```python
from build123d import *

# Parameters (mm, degrees)
SKETCH1_W           = 120
SKETCH1_H           = 120
BOSS_EXTRUDE1_DEPTH = 60
SHELL1_T            = -2
FILLET1_R           = 2
CUT_EXTRUDE1_REACH  = 148.969
SKETCH2_W           = 15
SKETCH2_H           = 15


with BuildPart() as part:
    # Sketch1 → Boss-Extrude1 (new body)
    with BuildSketch(Plane(origin=(0, 0, 0), x_dir=(1, 0, 0), z_dir=(0, 1, 0))):
        Rectangle(SKETCH1_W, SKETCH1_H)
    extrude(amount=BOSS_EXTRUDE1_DEPTH)

    # Shell1
    shell1_openings = [part.faces().sort_by_distance(p)[0] for p in [
        (0, 60, 0),
    ]]
    offset(amount=SHELL1_T, openings=shell1_openings, kind=Kind.INTERSECTION)

    # Fillet1
    fillet1_edges = [part.edges().sort_by_distance(p)[0] for p in [
        (0, 0, 60),
        (-60, 0, 0),
        (0, 0, -60),
        (60, 0, 0),
        (60, 30, 60),
        (-60, 30, 60),
        (-60, 30, -60),
        (60, 30, -60),
    ]]
    fillet(fillet1_edges, radius=FILLET1_R)

    # Sketch2 → Cut-Extrude1 (cut, up to next)
    with BuildSketch(Plane.XY.offset(60), mode=Mode.PRIVATE) as cut_extrude1_sk1:
        with Locations((-12.5, 25)):
            Rectangle(SKETCH2_W, SKETCH2_H)
    cut_extrude1_tool1 = extrude(cut_extrude1_sk1.sketch, amount=-CUT_EXTRUDE1_REACH, mode=Mode.PRIVATE) & part.part
    # Sketch2 → Cut-Extrude1 (cut, up to next)
    with BuildSketch(Plane.XY.offset(60), mode=Mode.PRIVATE) as cut_extrude1_sk2:
        with Locations((12.5, 25)):
            Rectangle(SKETCH2_W, SKETCH2_H)
    cut_extrude1_tool2 = extrude(cut_extrude1_sk2.sketch, amount=-CUT_EXTRUDE1_REACH, mode=Mode.PRIVATE) & part.part
    add(cut_extrude1_tool1.solids().sort_by_distance((-12.5, 25, 60))[0], mode=Mode.SUBTRACT)
    add(cut_extrude1_tool2.solids().sort_by_distance((12.5, 25, 60))[0], mode=Mode.SUBTRACT)


solid = part.part
```
Part model, mm, in its own coordinate system. A direction names the side the tool comes from. Round coordinates to 2 decimals unless told otherwise and drop trailing zeros. Loops run counter-clockwise (first coordinate to the right, second up) from the corner with the lowest first, then second, coordinate; pieces in that order, holes last. Notation, with made-up numbers: (20, 21.25) -> (52, 21.25) arc R10 cw to (52, 27.25) -> close; hole circle Ø10 at (61, 44). An arc over 180 degrees is marked (long way). Use a Markdown table: item, result.
1) Cut at A-A, the plane y = 40.5. List the corners of the cut face in (x, z), and give its area (3 significant figures).
The answers:
| item | result |
|---|---|
| outline | (-60, -58) arc R2 ccw to (-58, -60) -> (58, -60) arc R2 ccw to (60, -58) -> (60, 58) arc R2 ccw to (58, 60) -> (-58, 60) arc R2 ccw to (-60, 58) -> close; hole (-58, -58) -> (58, -58) -> (58, 58) -> (-58, 58) -> close |
| area | 941 mm2 |
2) Drop flat-ended pins along their axis: pin 1 Ø4 at (x, z) = (-32, -5.5) entering from +Y; pin 2 Ø1 at (x, y) = (11.5, 23.5) entering from +Z; pin 3 Ø0.6 at (x, z) = (-15.5, 59) entering from -Y. Give the stop position or say it passes through.
The answers:
| item | result |
|---|---|
| pin 1 | stops at y = 2 |
| pin 2 | stops at z = -58 |
| pin 3 | stops at y = 0.13 |
3) Cut at B-B, the plane x = -18. List the corners of the cut face in (y, z).
The answers:
| item | result |
|---|---|
| outline | (0, -58) arc R2 ccw to (2, -60) -> (60, -60) -> (60, -58) -> (2, -58) -> (2, 58) -> (17.5, 58) -> (17.5, 60) -> (2, 60) arc R2 ccw to (0, 58) -> close; (32.5, 58) -> (60, 58) -> (60, 60) -> (32.5, 60) -> close |
4) Pull direction Z, two halves, no side cores. Call faces 3 (the flat face through (-1, 31, -60)), 4 (the flat face through (-1, 2, -1)), 5 (the flat face through (-60, 31, 1)), 6 (the flat face through (-1, 31, 60)): pulls with the +Z half, pulls with the -Z half, needs draft (parallel to the pull), parting line crosses it, or undercut.
The answers:
| item | result |
|---|---|
| face 3 | pulls with the -Z half |
| face 4 | undercut |
| face 5 | needs draft |
| face 6 | pulls with the +Z half |
5) Cut at C-C, the plane x = -49. List the corners of the cut face in (y, z).
The answers:
| item | result |
|---|---|
| outline | (0, -58) arc R2 ccw to (2, -60) -> (60, -60) -> (60, -58) -> (2, -58) -> (2, 58) -> (60, 58) -> (60, 60) -> (2, 60) arc R2 ccw to (0, 58) -> close |
6) Probe line 1 (X direction, y = 35.5, z = 46); line 2 (Y direction, x = 28, z = 31). List the from-to ranges inside material, lowest first. Write a range as [from, to].
The answers:
| item | result |
|---|---|
| line 1 | x = [-60, -58], [58, 60] |
| line 2 | y = [0, 2] |
7) Tool access for faces 1 (the flat face through (-1, 0, -1)), 2 (the flat face through (-1, 31, 58)): list every direction of +Z, -Z, +X, -X, +Y, -Y with a clear straight run to the whole face (end or side of a thin tool).
The answers:
| item | result |
|---|---|
| face 1 | +Z, -Z, +X, -X, -Y |
| face 2 | +Y |
8) Cut at D-D, the plane z = 38.5. List the corners of the cut face in (x, y).
The answers:
| item | result |
|---|---|
| outline | (-60, 2) arc R2 ccw to (-58, 0) -> (58, 0) arc R2 ccw to (60, 2) -> (60, 60) -> (58, 60) -> (58, 2) -> (-58, 2) -> (-58, 60) -> (-60, 60) -> close |
